```python
from build123d import *

# Parameters (mm, degrees)
SKETCH1_R           = 64
SKETCH1_R_2         = 59
BOSS_EXTRUDE1_DEPTH = 27
SKETCH2_W           = 14
SKETCH2_H           = 59.5
CUT_EXTRUDE1_DEPTH  = 25
CIRPATTERN1_COUNT   = 16
SKETCH3_R           = 1.5
CUT_EXTRUDE2_DEPTH  = 28
CIRPATTERN2_COUNT   = 4


with BuildPart() as part:
    # Sketch1 → Boss-Extrude1 (new body)
    with BuildSketch(Plane(origin=(0, 0, 0), x_dir=(0, 0, -1), z_dir=(1, 0, 0))):
        Circle(SKETCH1_R)
        Circle(SKETCH1_R_2, mode=Mode.SUBTRACT)
    extrude(amount=BOSS_EXTRUDE1_DEPTH)

    # Sketch2 → Cut-Extrude1 (cut)
    with BuildSketch(Plane.ZY):
        with Locations((0, 29.75)):
            Rectangle(SKETCH2_W, SKETCH2_H)
    cut_extrude1 = extrude(amount=-CUT_EXTRUDE1_DEPTH, mode=Mode.SUBTRACT)

    # CirPattern1: Cut-Extrude1 ×16 about axis
    cirpattern1_axis = Axis((0, 0, 0), (1, 0, 0))
    for i in range(1, CIRPATTERN1_COUNT):
        add(cut_extrude1.rotate(cirpattern1_axis, i * 360 / CIRPATTERN1_COUNT), mode=Mode.SUBTRACT)

    # Sketch3 → Cut-Extrude2 (cut, through all)
    with BuildSketch(Plane.ZY):
        with Locations((11.998054804, 60.318294745)):
            Circle(SKETCH3_R)
    cut_extrude2 = extrude(amount=-CUT_EXTRUDE2_DEPTH, mode=Mode.SUBTRACT)

    # CirPattern2: Cut-Extrude2 ×4 about axis
    cirpattern2_axis = Axis((0, 0, 0), (1, 0, 0))
    for i in range(1, CIRPATTERN2_COUNT):
        add(cut_extrude2.rotate(cirpattern2_axis, i * 360 / CIRPATTERN2_COUNT), mode=Mode.SUBTRACT)


solid = part.part
```
Verification items for the finished model (mm, model axes). A direction names the side the tool comes from. Give positions to 0.01 mm unless a question says otherwise; leave off trailing zeros. Loops run counter-clockwise (first coordinate to the right, second up) from the corner with the lowest first, then second, coordinate; pieces in that order, holes last. Notation, with made-up numbers: M 13.5,14 L 54.5,14 A21 ccw 54.5,42 Z; hole C -10,-33.75 d3. An arc over 180 degrees is marked long. Return JSON: item names as keys, results as strings.
1) Tool access check on faces 4 (the flat face through (25, 41.8, -41.9)), 5 (the cylindrical face through (13.311, -12.69, 58.988)). Record the directions out of +Z, -Z, +X, -X, +Y, -Y that give a thin tool (end or side, any length) a straight path to the whole face; none if there is none.
Findings:
{"face 4": "-X", "face 5": "+X, -X"}
2) Section check D-D, the plane x = 10. Count the separate pieces of the cut face and the enclosed holes in it, and give its area (3 significant figures).
Findings:
{"separate pieces": "1", "enclosed holes": "5", "area": "1,760 mm2"}
3) Section check C-C, the plane y = -33. Enter the section's corners in (x, z), and give its area (3 significant figures).
Findings:
{"outline": "M 0,-54.84 L 27,-54.84 L 27,-48.91 L 0,-48.91 Z; M 0,48.91 L 27,48.91 L 27,54.84 L 0,54.84 Z", "area": "320 mm2"}
4) Material ranges on L1, parallel to Y at x = 8, z = -12; L2, parallel to Y at x = 9.75, z = -59; L3, parallel to Y at x = 22.5, z = -23, recorded low to high. Write a range as [from, to].
Findings:
{"L1": "y = [-62.86, -61.82], [-58.82, -57.77], [57.77, 62.86]", "L2": "y = [-24.8, -7], [7, 11.28], [12.71, 24.8]", "L3": "y = [-59.72, -54.88], [54.88, 59.72]"}
5) Section check A-A, the plane z = 0. Enter the section's corners in (x, y), and give its area (3 significant figures).
Findings:
{"outline": "M 0,-64 L 27,-64 L 27,-59 L 25,-59 L 25,-59.5 L 0,-59.5 Z; M 0,59.5 L 25,59.5 L 25,59 L 27,59 L 27,64 L 0,64 Z", "area": "245 mm2"}
6) Mould release check, pull along Y, two halves, no side actions. Record for faces 1 (the flat face through (12.3, -22.7, 55)), 2 (the flat face through (0, -57, 19)), 3 (the cylindrical face through (13.311, -58.988, -12.69)): released by +Y, released by -Y, zero draft, split by the parting line, or undercut.
Findings:
{"face 1": "undercut", "face 2": "zero draft", "face 3": "undercut"}
7) Gauge pin test, flat ends, axial feed: P1, Ø3, axis at x = 16.5, y = 13.5, coming from the -Z side; P2, Ø1, axis at x = 9, y = -59, coming from the +Z side; P3, Ø0.5, axis at x = 7, y = 59, coming from the -Z side. Record the tip position at first contact, or that the pin passes through.
Findings:
{"P1": "stops at z = -62.86", "P2": "stops at z = 25.96", "P3": "stops at z = -25.39"}
